Study the drawing (mm; zero at the part's minimum x, y, z) and answer. Coordinates: 2 decimals unless noted, no trailing zeros. Loops run counter-clockwise (first coordinate to the right, second up) from the corner with the lowest first, then second, coordinate; pieces in that order, holes last.
Q1. A flat-ended cylindrical pin translates along its axis: P1, Ø12, axis at x = 143, y = 55.5, coming from the +Z side. Find the tip coordinate at first contact, or state that the pin passes through.
Q2. Straight lines are drawn through the part: line 1 (Y direction, x = 317, z = 1.25); line 2 (Y direction, x = 311.5, z = 4.5); line 3 (X direction, y = 120, z = 6.75). For each, find the intervals that lie inside material, in ascending order.
Q3. Section A-A (x = 260.5) is taken. Give the vertices of the cut face in (y, z), then the cut area to 3 significant figures.
Q4. Section D-D (y = 49) is taken. Give the vertices of the cut face in (x, z).
Q5. Section C-C (x = 343) is taken. Give the vertices of the cut face in (y, z).
Q6. Section B-B (z = 5.5) is taken. Give the vertices of the cut face in (x, y), then the cut area to 3 significant figures.
Q7. The mould has two halves that part along Y. Classify the marked faces 1 and 2: pulls with the +Y half, pulls with the -Y half, needs draft (parallel to the pull), parting line crosses it, or undercut.
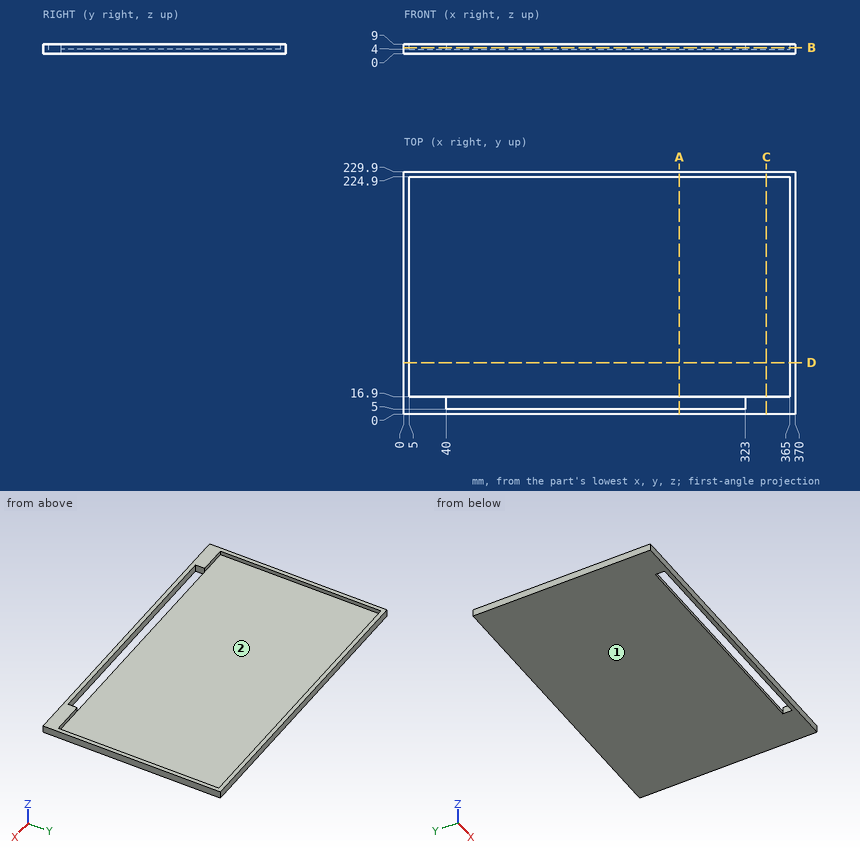
Numbers:
1. P1: stops at z = 4
2. line 1: y = 0 to 5, 16.9 to 229.9
2. line 2: y = 0 to 5, 224.9 to 229.9
2. line 3: x = 0 to 5, 365 to 370
3. outline: (0, 0) - (5, 0) - (5, 9) - (0, 9) - close; (16.9, 0) - (229.9, 0) - (229.9, 9) - (224.9, 9) - (224.9, 4) - (16.9, 4) - close
3. area: 922 mm2
4. outline: (0, 0) - (370, 0) - (370, 9) - (365, 9) - (365, 4) - (5, 4) - (5, 9) - (0, 9) - close
5. outline: (0, 0) - (229.9, 0) - (229.9, 9) - (224.9, 9) - (224.9, 4) - (16.9, 4) - (16.9, 9) - (0, 9) - close
6. outline: (0, 0) - (370, 0) - (370, 229.9) - (0, 229.9) - close; hole (5, 16.9) - (40, 16.9) - (40, 5) - (323, 5) - (323, 16.9) - (365, 16.9) - (365, 224.9) - (5, 224.9) - close
6. area: 6,820 mm2
7. face 1: needs draft
7. face 2: undercut
